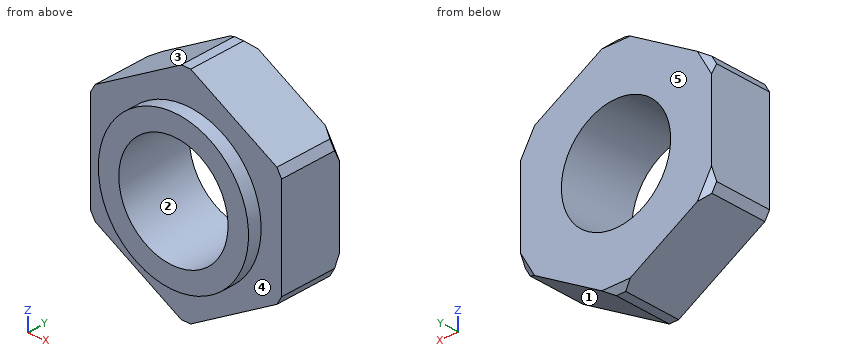
Autodesk Inventor part; units mm, degrees
ref_plane "YZ Plane" through (0, 0, 0) normal (1, 0, 0) x (0, 1, 0)
ref_plane "XZ Plane" through (0, 0, 0) normal (0, 1, 0) x (-1, 0, 0)
ref_plane "XY Plane" through (0, 0, 0) normal (0, 0, 1) x (1, 0, 0)
sketch "スケッチ2" plane through (0, 0, 0) normal (0, 1, 0) x (-1, 0, 0)
  circle A0 centre (0, 0) radius 2
  circle A1 centre (0, 0) radius 2.75
  circle A2 centre (0, 0) radius 3.5
  line L0 (3.2709, 0) -> (-4.3069, 0) construction
  line L1 (-3.5, -2.0207) -> (0, -4.0415)
  line L2 (-3.5, 0) -> (-3.5, -2.0207)
  line L3 (0, 3.4516) -> (0, -4.8702) construction
  line L4 (-3.5, 2.0207) -> (0, 4.0415)
  line L5 (-3.5, 0) -> (-3.5, 2.0207)
  line L6 (3.5, -2.0207) -> (0, -4.0415)
  line L7 (3.5, 0) -> (3.5, -2.0207)
  line L8 (3.5, 2.0207) -> (0, 4.0415)
  line L9 (3.5, 0) -> (3.5, 2.0207)
  dimension "d8" = 7
  dimension "d6" = 4
  dimension "d7" = 5.5
  dimension "d25" = 120
extrude "押し出し1" add sketch "スケッチ2" against normal blind 0.5 contours A1
extrude "押し出し2" add sketch "スケッチ2" along normal blind 2.3 contours A1 | A2 | L7 L6 A2 | A2 L8 L9 | A2 L4 L8 | L6 L1 A2 | A2 L5 L4 | L1 L2 A2
chamfer "面取り1" distance 0.2 angle 45 6 edges at (3.5, 1.15, -2.0207) (0, 1.15, -4.0415) (-3.5, 1.15, -2.0207) (-3.5, 1.15, 2.0207) (0, 1.15, 4.0415) (3.5, 1.15, 2.0207)
chamfer "面取り2" distance 0.2 angle 45 6 edges at (3.4134, 2.3, -1.9707) (0, 2.3, -3.9415) (-3.4134, 2.3, -1.9707) (-3.4134, 2.3, 1.9707) (0, 2.3, 3.9415) (3.4134, 2.3, 1.9707)
thread "ねじ1"
properties part number "S4-05-3W" material "ステンレス鋼 AISI 304"
Geometry: final body of the model. Coordinates: model frame, mm. Face numbers are marked on the shaded views. A direction names the side the tool comes from. Round coordinates to 2 decimals unless told otherwise and drop trailing zeros. Loops run counter-clockwise (first coordinate to the right, second up) from the corner with the lowest first, then second, coordinate; pieces in that order, holes last. Notation, with made-up numbers: (15.5, -13.75) -> (49.5, -13.75) arc R20 cw to (49.5, 9.25) -> close; hole circle Ø4 at (-24, -5.5). An arc over 180 degrees is marked (long way). Write each question's results on one line, items separated by ' | '.
Item 1: Cut plane D-D on x = 0.75. Return the cut outline in (y, z).
Answers below:
outline: (-0.5, -2.65) -> (0, -2.65) -> (0, -3.61) -> (2.3, -3.61) -> (2.3, -1.85) -> (-0.5, -1.85) -> close; (-0.5, 1.85) -> (2.3, 1.85) -> (2.3, 3.61) -> (0, 3.61) -> (0, 2.65) -> (-0.5, 2.65) -> close
Item 2: Set-up query: the marked faces 4 and 5. Return all of +Z, -Z, +X, -X, +Y, -Y with unobstructed straight access to the full face (end or side cutting, diameter ignored); none if empty.
Answers below:
face 4: -Y | face 5: +Z, -Z, +X, -X, +Y
Item 3: Cut plane A-A on z = 0. Return the cut outline in (x, y), and give its area (3 significant figures).
Answers below:
outline: (-3.5, 0) -> (-2.75, 0) -> (-2.75, -0.5) -> (-2, -0.5) -> (-2, 2.3) -> (-3.5, 2.3) -> close; (2, -0.5) -> (2.75, -0.5) -> (2.75, 0) -> (3.5, 0) -> (3.5, 2.3) -> (2, 2.3) -> close | area: 7.65 mm²
Item 4: Pin query (flat end, axial travel): pin 1 Ø1.5 at (x, z) = (-0.5, 0) entering from +Y. Return the tip coordinate at first contact, or that it passes through.
Answers below:
pin 1: passes through
Item 5: Pull-direction query (X, two-part tool) for the marked faces 1, 2 and 3; classes: pulls with the +X half, pulls with the -X half, needs draft (parallel to the pull), parting line crosses it, or undercut.
Answers below:
face 1: pulls with the +X half | face 2: undercut | face 3: pulls with the -X half
Item 6: Cut plane B-B on x = 0. Return the cut outline in (y, z).
Answers below:
outline: (-0.5, -2.75) -> (0, -2.75) -> (0, -3.94) -> (2.1, -3.94) -> (2.3, -3.74) -> (2.3, -2) -> (-0.5, -2) -> close; (-0.5, 2) -> (2.3, 2) -> (2.3, 3.74) -> (2.1, 3.94) -> (0, 3.94) -> (0, 2.75) -> (-0.5, 2.75) -> close
Item 7: Line query: probe 1 along Z at (x, y) = (0, 0.8); probe 2 along X at (y, z) = (1.1, -0.75); probe 3 along Y at (x, z) = (2.25, -1.75). Output: solid intervals per line, ascending. Write a range as [from, to].
Answers below:
probe 1: z = [-3.94, -2], [2, 3.94] | probe 2: x = [-3.5, -1.85], [1.85, 3.5] | probe 3: y = [0, 2.3]
Item 8: Cut plane C-C on y = 1.8. Return the cut outline in (x, z), and give its area (3 significant figures).
Answers below:
outline: (-3.5, -1.82) -> (-3.33, -2.12) -> (-0.17, -3.94) -> (0.17, -3.94) -> (3.33, -2.12) -> (3.5, -1.82) -> (3.5, 1.82) -> (3.33, 2.12) -> (0.17, 3.94) -> (-0.17, 3.94) -> (-3.33, 2.12) -> (-3.5, 1.82) -> close; hole circle Ø4 at (0, 0) | area: 29.8 mm²
